from build123d import *

# Parameters (mm, degrees)
SKETCH1_R           = 4.5
BOSS_EXTRUDE1_DEPTH = 1.57
SKETCH2_R           = 2
BOSS_EXTRUDE2_DEPTH = 5.1
SKETCH5_W           = 1.2
SKETCH5_H           = 0.798080121
SKETCH4_R           = 4
BOSS_EXTRUDE3_DEPTH = 0.65


with BuildPart() as part:
    # Sketch1 → Boss-Extrude1 (new body)
    with BuildSketch(Plane(origin=(0, 0, 0), x_dir=(1, 0, 0), z_dir=(0, 1, 0))):
        with Locations(Location((0, 0, 0), (0, 0, 270))):
            Circle(SKETCH1_R)
    extrude(amount=BOSS_EXTRUDE1_DEPTH)

    # Sketch2 → Boss-Extrude2 (add)
    with BuildSketch(Plane(origin=(0, 1.57, 0), x_dir=(1, 0, 0), z_dir=(0, 1, 0))):
        with Locations(Location((0, 0, 0), (0, 0, 270))):
            Circle(SKETCH2_R)
    extrude(amount=BOSS_EXTRUDE2_DEPTH)

    # Sketch3 → Revolve1 (revolve)
    with BuildSketch(Plane(origin=(0, 6.67, 0), x_dir=(1, 0, 0), z_dir=(0, 1, 0))):
        with BuildLine():
            Line((0, 4.75), (0, -4.75))
            ThreePointArc((0, -4.75), (4.75, 0), (0, 4.75))
        make_face()
    revolve(axis=Axis((0, 6.67, -8.311953328), (0, 0, 1)))

    # Sketch5 → Cut-Revolve1 (revolve, cut)
    with BuildSketch(Plane.XY, mode=Mode.PRIVATE) as cut_revolve1_sk:
        with Locations((2.6, 2.760618076)):
            Rectangle(SKETCH5_W, SKETCH5_H)
    revolve(cut_revolve1_sk.sketch.rotate(Axis((0, 3.159658136, 0), (0, -1, 0)), 90), axis=Axis((0, 3.159658136, 0), (0, -1, 0)), mode=Mode.SUBTRACT)

    # Sketch4 → Boss-Extrude3 (add)
    with BuildSketch(Plane.XZ):
        with Locations(Location((0, 0, 0), (0, 0, 270))):
            Circle(SKETCH4_R)
    extrude(amount=BOSS_EXTRUDE3_DEPTH)


solid = part.part
The listing builds one solid part. Answer for the finished solid, in the listing's coordinates (mm). A direction names the side the tool comes from. Round coordinates to 2 decimals unless told otherwise and drop trailing zeros. Write each loop counter-clockwise with the first axis right and the second up, starting at its lowest first coordinate (ties: lowest second). Pieces come first, ordered by that corner, then holes. Notation, with made-up numbers: M 18.25,-9 L 54.25,-9 A31 cw 54.25,25 Z; hole C -10,33 d8. An arc over 180 degrees is marked long. Write each question's results on one line, items separated by ' | '. Start each with the question number.
Item 1: Given pin 1 Ø5 at (y, z) = (7.5, 2.5) entering from -X; pin 2 Ø1.5 at (x, z) = (-0.5, -1.5) entering from +Y; pin 3 Ø1.5 at (x, y) = (3.5, 7) entering from +Z, each flat-ended and moving along its own axis, determine where each tip first touches the part or whether it passes through.
Item 2: Find section B-B on x = 0. Write down the section's boundary in (y, z).
Item 3: Which of the six approach directions +Z, -Z, +X, -X, +Y, -Y give full straight-line access (tool end or side, diameter ignored) to faces 1 (the flat face through (0, -0.65, 0)), 2 (the cylindrical face through (-3.905, -0.32, 0.867))?
Item 4: Find section C-C on z = 0. Write down the section's boundary in (x, y), and give its area (3 significant figures).
Item 5: Find section A-A on z = 2.5. Write down the section's boundary in (x, y), and give its area (3 significant figures).
Item 6: Straight lines are drawn through the part: probe 1 along X at (y, z) = (8.75, -1.5); probe 2 along Y at (x, z) = (2, 3); probe 3 along Y at (x, z) = (2.5, -3.5). For each, find the intervals that lie inside material, in ascending order.
Item 7: Find section D-D on y = 8. Write down the section's boundary in (x, z).
Item 8: The mould has two halves that part along Y. Classify faces 3 (the flat face through (1, 3.16, -2)), 4 (the flat face through (-3, 0, -3)), 5 (the cylindrical face through (1.352, 0.774, 4.292)), 6 (the flat face through (-1, 1.57, 2)): +Y half, -Y half, draft (parallel to the pull), parting line (faces both ways), or undercut.
Answer block:
1) pin 1: stops at x = -4.75 | pin 2: stops at y = 11.35 | pin 3: stops at z = 3.86
2) outline: M -0.65,-4 L 0,-4 L 0,-4.5 L 1.57,-4.5 L 1.57,-2 L 3.16,-2 L 3.16,-3.2 A4.75 ccw long 3.16,3.2 L 3.16,2 L 1.57,2 L 1.57,4.5 L 0,4.5 L 0,4 L -0.65,4 Z
3) face 1: +Z, -Z, +X, -X, -Y | face 2: -Y
4) outline: M -4.5,0 L -4,0 L -4,-0.65 L 4,-0.65 L 4,0 L 4.5,0 L 4.5,1.57 L 2,1.57 L 2,3.16 L 3.2,3.16 A4.75 ccw long -3.2,3.16 L -2,3.16 L -2,1.57 L -4.5,1.57 Z | area: 91.1 mm²
5) outline: M -3.74,0 L -3.12,0 L -3.12,-0.65 L 3.12,-0.65 L 3.12,0 L 3.74,0 L 3.74,1.57 L -3.74,1.57 Z; M -2,3.16 L 2,3.16 A4.04 ccw long Z | area: 65.6 mm²
6) probe 1: x = -4 to 4 | probe 2: y = -0.65 to 1.57, 3.58 to 9.76 | probe 3: y = 0 to 1.57, 4.65 to 8.69
7) outline: C 0,0 d9.12
8) face 3: undercut | face 4: -Y half | face 5: draft | face 6: undercut
